Could you check a few things on this model? Use its own coordinates, in mm. Face numbers are marked on the shaded views. A direction names the side the tool comes from. Give positions to 0.01 mm unless a question says otherwise; leave off trailing zeros. Order: outer loops, then holes, each group sorted by start corner. A loop starts at its lowest first (then second) coordinate and runs counter-clockwise, first axis right, second up.
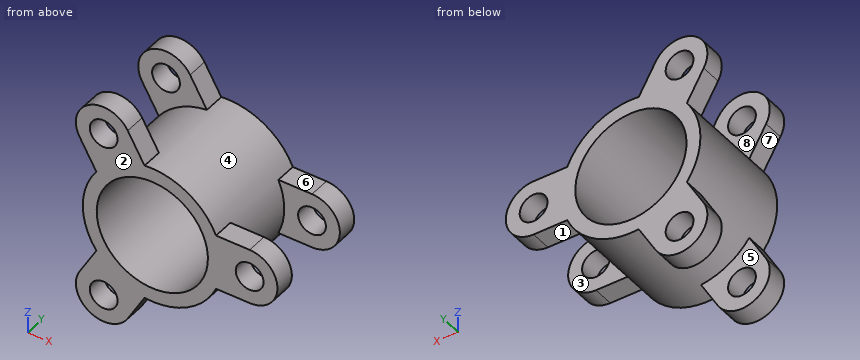
from build123d import *

# Parameters (mm, degrees)
SKETCH1_R           = 50
SKETCH1_R_2         = 40
BOSS_EXTRUDE2_DEPTH = 80
SKETCH1_4_R         = 10
BOSS_EXTRUDE4_DEPTH = 15


with BuildPart() as part:
    # Sketch1 → Boss-Extrude2 (new body)
    with BuildSketch(Plane(origin=(0, 0, 0), x_dir=(1, 0, 0), z_dir=(0, 1, 0))):
        with Locations(Location((0, 0, 0), (0, 0, 270))):
            Circle(SKETCH1_R)
        with Locations(Location((0, 0, 0), (0, 0, 270))):
            Circle(SKETCH1_R_2, mode=Mode.SUBTRACT)
    extrude(amount=BOSS_EXTRUDE2_DEPTH)

    # Sketch1_4 → Boss-Extrude4 (add)
    # profile 1 of 3: a face of its own
    with BuildSketch(Plane(origin=(0, 0, 0), x_dir=(1, 0, 0), z_dir=(0, 1, 0))):
        with BuildLine():
            Line((-17.679491924, -70.621778265), (-5.592370399, -49.686269666))
            ThreePointArc((-5.592370399, -49.686269666), (-25, -43.301270189), (-40.23338655, -29.686269666))
            Line((-40.23338655, -29.686269666), (-52.320508076, -50.621778265))
            ThreePointArc((-52.320508076, -50.621778265), (-45, -77.942286341), (-17.679491924, -70.621778265))
        make_face()
        with Locations(Location((-35, -60.621778265, 0), (0, 0, 270))):
            Circle(SKETCH1_4_R, mode=Mode.SUBTRACT)
    # profile 2 of 3: a face of its own
    with BuildSketch(Plane(origin=(0, 0, 0), x_dir=(1, 0, 0), z_dir=(0, 1, 0))):
        with BuildLine():
            ThreePointArc((-40.23338655, 29.686269666), (-25, 43.301270189), (-5.592370399, 49.686269666))
            Line((-5.592370399, 49.686269666), (-17.679491924, 70.621778265))
            ThreePointArc((-17.679491924, 70.621778265), (-45, 77.942286341), (-52.320508076, 50.621778265))
            Line((-52.320508076, 50.621778265), (-40.23338655, 29.686269666))
        make_face()
        with Locations(Location((-35, 60.621778265, 0), (0, 0, 270))):
            Circle(SKETCH1_4_R, mode=Mode.SUBTRACT)
    # profile 3 of 3: a face of its own
    with BuildSketch(Plane(origin=(0, 0, 0), x_dir=(1, 0, 0), z_dir=(0, 1, 0))):
        with BuildLine():
            ThreePointArc((70, -20), (90, 0), (70, 20))
            Line((70, 20), (45.82575695, 20))
            ThreePointArc((45.82575695, 20), (48.945315647, 10.215482184), (50, 0))
            ThreePointArc((50, 0), (48.945315647, -10.215482184), (45.82575695, -20))
            Line((45.82575695, -20), (70, -20))
        make_face()
        with Locations(Location((70, 0, 0), (0, 0, 270))):
            Circle(SKETCH1_4_R, mode=Mode.SUBTRACT)
    boss_extrude4 = extrude(amount=BOSS_EXTRUDE4_DEPTH)

    # Mirror1: Boss-Extrude4 across plane
    add(boss_extrude4.mirror(Plane.ZX.offset(40)))


solid = part.part
Item 1: We'd pull the mould along Y, two halves only. Please class the marked faces 1, 2 and 3: +Y half, -Y half, draft (parallel to the pull), parting line (faces both ways), or undercut.
Findings:
face 1: draft
face 2: -Y half
face 3: undercut
Item 2: Please list where these lines run through material, in increasing order: line 1 along Z through (x, y) = (-1, 4); line 2 along Z through (x, y) = (21, 4.5); line 3 along X through (y, z) = (62, -30.5).
Findings:
line 1: z = -49.99 to -39.99, 39.99 to 49.99
line 2: z = -45.38 to -34.04, 34.04 to 45.38
line 3: x = -39.62 to -25.88, 25.88 to 39.62
Item 3: Imagine slicing it at C-C on y = 12. List the corners of the cut face in (x, z) for me, then the cut area to 3 significant figures.
Findings:
outline: (-52.32, -50.62) arc R20 ccw to (-17.68, -70.62) - (-5.59, -49.69) arc R50 ccw to (45.83, -20) - (70, -20) arc R20 ccw to (70, 20) - (45.83, 20) arc R50 ccw to (-5.59, 49.69) - (-17.68, 70.62) arc R20 ccw to (-52.32, 50.62) - (-40.23, 29.69) arc R50 ccw to (-40.23, -29.69) - close; hole circle Ø20 at (-35, -60.62); hole circle Ø20 at (-35, 60.62); hole circle Ø80 at (0, 0); hole circle Ø20 at (70, 0)
area: 6,330 mm2
Item 4: Imagine slicing it at B-B on x = 0. List the corners of the cut face in (y, z) for me.
Findings:
outline: (0, -50) - (80, -50) - (80, -40) - (0, -40) - close; (0, 40) - (80, 40) - (80, 50) - (0, 50) - close
Item 5: Imagine slicing it at D-D on x = -35. Give the number of separate pieces and of enclosed holes in the cut face, then the cut area to 3 significant figures.
Findings:
separate pieces: 6
enclosed holes: 0
area: 4,110 mm2
Item 6: Imagine slicing it at A-A on z = 0. List the corners of the cut face in (x, y) for me.
Findings:
outline: (-50, 0) - (-40, 0) - (-40, 80) - (-50, 80) - close; (40, 0) - (60, 0) - (60, 15) - (50, 15) - (50, 65) - (60, 65) - (60, 80) - (40, 80) - close; (80, 0) - (90, 0) - (90, 15) - (80, 15) - close; (80, 65) - (90, 65) - (90, 80) - (80, 80) - close
Item 7: For the marked faces 4, 5, 6, 7 and 8, which set-ups out of +Z, -Z, +X, -X, +Y, -Y let a thin tool reach every point of the face, with its end or its side?
Findings:
face 4: none
face 5: -Z, -X
face 6: +Z, +X, +Y, -Y
face 7: -X, +Y, -Y
face 8: +Z, -X
Item 8: For pin 1 (4.5 mm diameter, centred on x = 60.5, y = 74, fed in from -Z); pin 2 (3 mm diameter, centred on x = 12.5, y = 39, fed in from +Z) (3 decimals); pin 3 (4.5 mm diameter, centred on x = 54, y = 74, fed in from +Z); pin 4 (18 mm diameter, centred on x = -35, z = 60.62, fed in from -Y), each with a flat end and sliding along its axis, tell me the tip position at first contact or that it passes through.
Findings:
pin 1: stops at z = -20
pin 2: stops at z = 48.775
pin 3: stops at z = 20
pin 4: passes through
